Work out the finished part from the listing and answer in its coordinate system (mm). Face numbers are marked on the shaded views. Round coordinates to 2 decimals unless told otherwise and drop trailing zeros. Write each loop counter-clockwise with the first axis right and the second up, starting at its lowest first coordinate (ties: lowest second). Pieces come first, ordered by that corner, then holes.
1. Find section A-A (x = 0). Write down the section's boundary in (y, z), and give its area (4 significant figures).
2. Find section D-D (y = -11.5). Write down the section's boundary in (x, z).
3. Flat-ended cylindrical pins translate along their axes: pin 1 Ø17 at (y, z) = (0, 25) entering from -X; pin 2 Ø13.5 at (x, z) = (0, 25) entering from -Y. Find the tip coordinate at first contact, or state that the pin passes through.
4. Find section B-B (z = 19). Write down the section's boundary in (x, y).
5. Straight lines are drawn through the part: probe 1 along Z at (x, y) = (0, 13); probe 2 along Y at (x, z) = (0, 42); probe 3 along X at (y, z) = (-0.5, 47.5). For each, find the intervals that lie inside material, in ascending order.
6. Determine the mould class of the marked faces 1, 2 and 3 for opening direction Y: pulls with the +Y half, pulls with the -Y half, needs draft (parallel to the pull), parting line crosses it, or undercut.
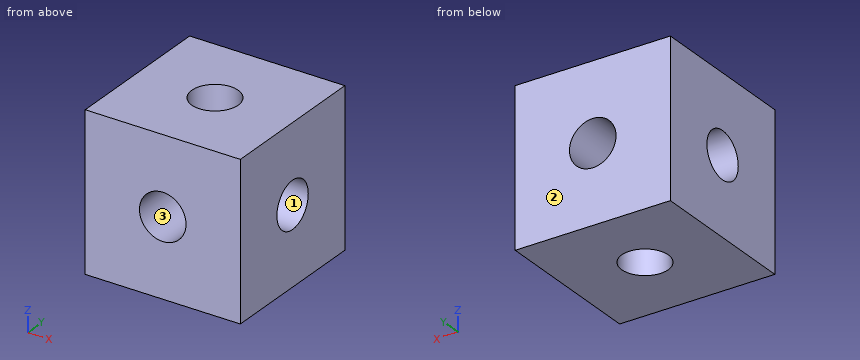
```python
from build123d import *

# Parameters (mm, degrees)
F0_W      = 50
F0_H      = 50
F1_DEPTH  = 50
F2_R      = 7.5
F8_DEPTH  = 25
F3_R      = 7.5
F9_DEPTH  = 25
F4_R      = 7.5
F10_DEPTH = 25
F5_R      = 7.5
F11_DEPTH = 25
F6_R      = 7.5
F12_DEPTH = 25
F7_R      = 7.5
F13_DEPTH = 25


with BuildPart() as f1:
    # F0 (on Top) → F1 (new body)
    with BuildSketch(Plane.XY):
        Rectangle(F0_W, F0_H)
    extrude(amount=F1_DEPTH)

    # F2 (on face) → F8 (cut)
    with BuildSketch(Plane.XY.offset(50)):
        Circle(F2_R)
    extrude(amount=-F8_DEPTH, mode=Mode.SUBTRACT)

    # F3 (on face) → F9 (cut)
    with BuildSketch(Plane(origin=(0, 25, 0), x_dir=(-1, 0, 0), z_dir=(0, 1, 0))):
        with Locations((0, 25)):
            Circle(F3_R)
    extrude(amount=-F9_DEPTH, mode=Mode.SUBTRACT)

    # F4 (on face) → F10 (cut)
    with BuildSketch(Plane.XZ.offset(25)):
        with Locations((0, 25)):
            Circle(F4_R)
    extrude(amount=-F10_DEPTH, mode=Mode.SUBTRACT)

    # F5 (on face) → F11 (cut)
    with BuildSketch(Plane(origin=(-25, 0, 0), x_dir=(0, -1, 0), z_dir=(-1, 0, 0))):
        with Locations((0, 25)):
            Circle(F5_R)
    extrude(amount=-F11_DEPTH, mode=Mode.SUBTRACT)

    # F6 (on face) → F12 (cut)
    with BuildSketch(Plane.YZ.offset(25)):
        with Locations((0, 25)):
            Circle(F6_R)
    extrude(amount=-F12_DEPTH, mode=Mode.SUBTRACT)

    # F7 (on face) → F13 (cut)
    with BuildSketch(Plane.XY):
        Circle(F7_R)
    extrude(amount=F13_DEPTH, mode=Mode.SUBTRACT)


solid = f1.part
```
Worked answers:
1. outline: (-25, 0) - (-7.5, 0) - (-7.5, 17.5) - (-25, 17.5) - close; (-25, 32.5) - (-7.5, 32.5) - (-7.5, 50) - (-25, 50) - close; (7.5, 0) - (25, 0) - (25, 17.5) - (7.5, 17.5) - close; (7.5, 32.5) - (25, 32.5) - (25, 50) - (7.5, 50) - close
1. area: 1,225 mm2
2. outline: (-25, 0) - (25, 0) - (25, 50) - (-25, 50) - close; hole circle Ø15 at (0, 25)
3. pin 1: stops at x = -25
3. pin 2: passes through
4. outline: (-25, -25) - (-4.5, -25) - (-4.5, -6) arc R7.5 cw to (-6, -4.5) - (-25, -4.5) - close; (-25, 4.5) - (-6, 4.5) arc R7.5 cw to (-4.5, 6) - (-4.5, 25) - (-25, 25) - close; (4.5, -25) - (25, -25) - (25, -4.5) - (6, -4.5) arc R7.5 cw to (4.5, -6) - close; (4.5, 6) arc R7.5 cw to (6, 4.5) - (25, 4.5) - (25, 25) - (4.5, 25) - close
5. probe 1: z = 0 to 17.5, 32.5 to 50
5. probe 2: y = -25 to -7.5, 7.5 to 25
5. probe 3: x = -25 to -7.48, 7.48 to 25
6. face 1: undercut
6. face 2: pulls with the +Y half
6. face 3: needs draft
